Can you work these out from the drawing? Everything is in mm from the part's minimum corner. A direction names the side the tool comes from. Coordinates: 2 decimals unless noted, no trailing zeros. Loops run counter-clockwise (first coordinate to the right, second up) from the corner with the lowest first, then second, coordinate; pieces in that order, holes last. Notation, with made-up numbers: (8, -15.5) -> (40, -15.5) arc R15 ccw to (40, 7.5) -> close; hole circle Ø1 at (6.25, 25.25). An arc over 180 degrees is marked (long way). One line per question, with ' | ' between items.
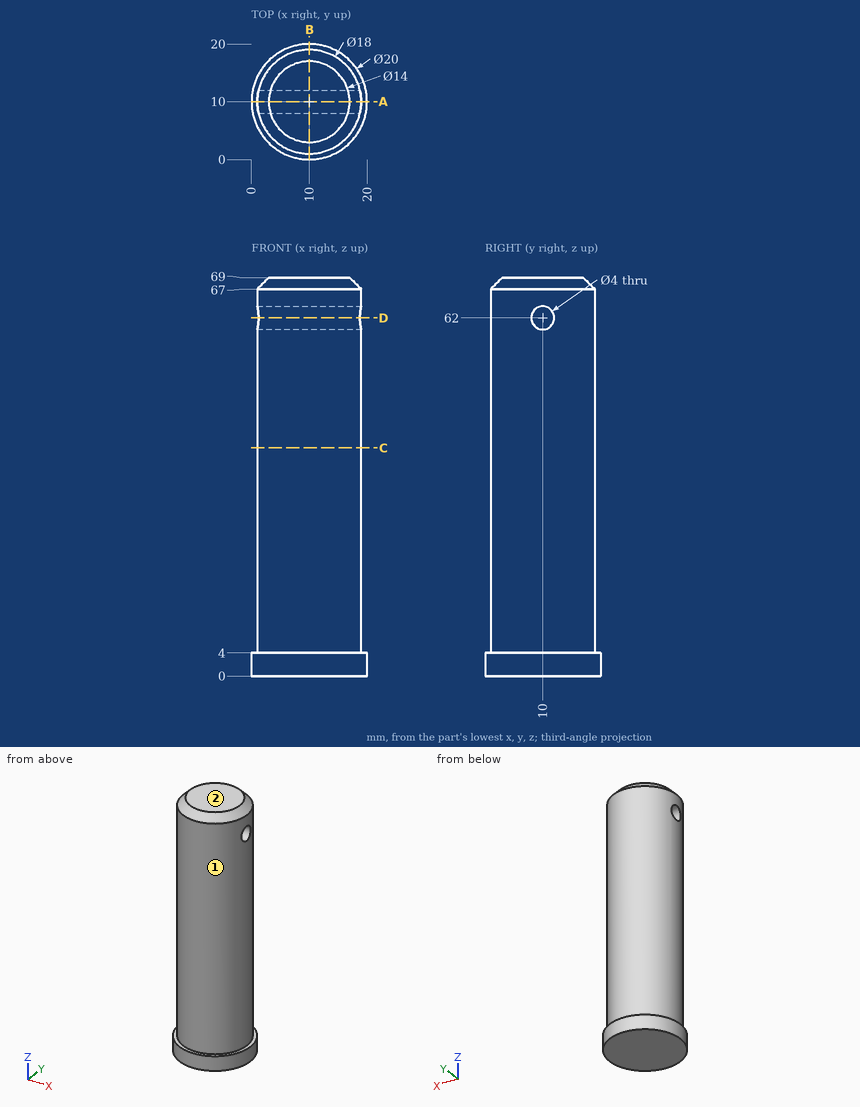
Q1. Please list where these lines run through material, in increasing order: L1, parallel to Z at x = 10.75, y = 10; L2, parallel to Y at x = 5.75, z = 62; L3, parallel to Z at x = 18, y = 11.25. Write a range as [from, to].
Values follow:
L1: z = [0, 60], [64, 69] | L2: y = [2.07, 8], [12, 17.93] | L3: z = [0, 60.44], [63.56, 67.9]
Q2. For pin 1 (6 mm diameter, centred on y = 16, z = 21, fed in from -X); pin 2 (1 mm diameter, centred on x = 14, z = 15, fed in from +Y); pin 3 (10 mm diameter, centred on x = 13.5, z = 40.5, fed in from +Y); pin 4 (6 mm diameter, centred on x = 14.5, y = 4.5, fed in from +Z), each with a flat end and sliding along its axis, tell me the tip position at first contact or that it passes through.
Values follow:
pin 1: stops at x = 1.51 | pin 2: stops at y = 18.29 | pin 3: stops at y = 19 | pin 4: stops at z = 69
Q3. Imagine slicing it at C-C on z = 39.5. Write out the boundary of the cut face in (x, y), plus the area to 3 significant figures.
Values follow:
outline: circle Ø18 at (10, 10) | area: 254 mm2
Q4. For the marked faces 1 and 2, which set-ups out of +Z, -Z, +X, -X, +Y, -Y let a thin tool reach every point of the face, with its end or its side?
Values follow:
face 1: +Z | face 2: +Z, +X, -X, +Y, -Y
Q5. Imagine slicing it at A-A on y = 10. Write out the boundary of the cut face in (x, z).
Values follow:
outline: (0, 0) -> (20, 0) -> (20, 4) -> (19, 4) -> (19, 60) -> (1, 60) -> (1, 4) -> (0, 4) -> close; (1, 64) -> (19, 64) -> (19, 67) -> (17, 69) -> (3, 69) -> (1, 67) -> close
Q6. Imagine slicing it at D-D on z = 62. Write out the boundary of the cut face in (x, y).
Values follow:
outline: (1.23, 8) arc R9 ccw to (18.77, 8) -> close; (1.23, 12) -> (18.77, 12) arc R9 ccw to start
Q7. Imagine slicing it at B-B on x = 10. Write out the boundary of the cut face in (y, z), plus the area to 3 significant figures.
Values follow:
outline: (0, 0) -> (20, 0) -> (20, 4) -> (19, 4) -> (19, 67) -> (17, 69) -> (3, 69) -> (1, 67) -> (1, 4) -> (0, 4) -> close; hole circle Ø4 at (10, 62) | area: 1,230 mm2
